```python
from build123d import *

# Parameters (mm, degrees)
F0_W     = 41
F0_H     = 41
F1_DEPTH = 4
F2_R     = 5


with BuildPart() as f1:
    # F0 (on Front) → F1 (new body)
    with BuildSketch(Plane.XZ):
        Rectangle(F0_W, F0_H)
        with BuildLine():
            ThreePointArc((-16, 14.3), (-17.202082, 17.202082), (-14.3, 16))
            Line((-14.3, 16), (-10.246951, 16))
            ThreePointArc((-10.246951, 16), (0, 19), (10.246951, 16))
            Line((10.246951, 16), (14.3, 16))
            ThreePointArc((14.3, 16), (16, 17.7), (17.7, 16))
            ThreePointArc((17.7, 16), (17.202082, 14.797918), (16, 14.3))
            Line((16, 14.3), (16, 10.246951))
            ThreePointArc((16, 10.246951), (18.234583, 5.338539), (19, 0))
            ThreePointArc((19, 0), (18.234583, -5.338539), (16, -10.246951))
            Line((16, -10.246951), (16, -14.3))
            ThreePointArc((16, -14.3), (17.202082, -14.797918), (17.7, -16))
            ThreePointArc((17.7, -16), (16, -17.7), (14.3, -16))
            Line((14.3, -16), (10.246951, -16))
            ThreePointArc((10.246951, -16), (0, -19), (-10.246951, -16))
            Line((-10.246951, -16), (-14.3, -16))
            ThreePointArc((-14.3, -16), (-17.202082, -17.202082), (-16, -14.3))
            Line((-16, -14.3), (-16, -10.246951))
            ThreePointArc((-16, -10.246951), (-19, 0), (-16, 10.246951))
            Line((-16, 10.246951), (-16, 14.3))
        make_face(mode=Mode.SUBTRACT)
    extrude(amount=F1_DEPTH)

    # F2
    f2_edges = [f1.edges().sort_by_distance(p)[0] for p in [
        (-20.5, -2, -20.5),
        (20.5, -2, -20.5),
        (20.5, -2, 20.5),
        (-20.5, -2, 20.5),
    ]]
    fillet(f2_edges, radius=F2_R)


solid = f1.part
```
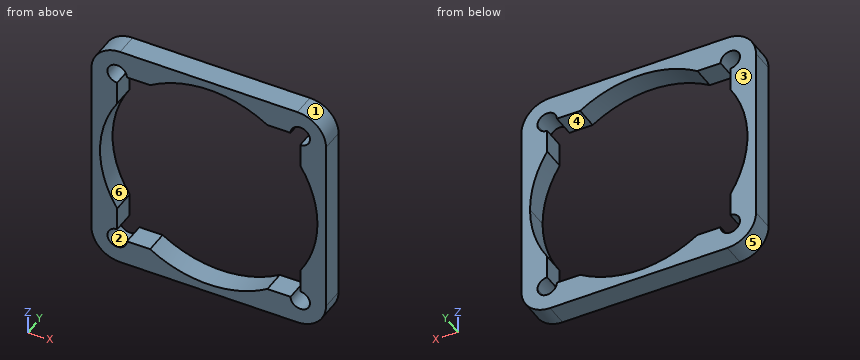
The model under review builds one solid part; all positions refer to its coordinate system, in mm. Face numbers are marked on the shaded views. A direction names the side the tool comes from. Round coordinates to 2 decimals unless told otherwise and drop trailing zeros. Write each loop counter-clockwise with the first axis right and the second up, starting at its lowest first coordinate (ties: lowest second). Pieces come first, ordered by that corner, then holes. Notation, with made-up numbers: M -30,-28 L -1,-28 A21 ccw -1,3 Z; hole C 43,-37 d3. An arc over 180 degrees is marked long. Use CSV: the item, a comma, the result in double quotes. Start each with the question number.
(1) We need section B-B, the plane x = -7.5. State the section outline as (y, z) points, then the cut area to 3 significant figures.
(2) Tool access review of the marked faces 5 and 6: name each direction out of +Z, -Z, +X, -X, +Y, -Y from which nothing blocks a thin tool from reaching the whole face with its end or side.
(3) We need section C-C, the plane z = 4. State the section outline as (x, y) points.
(4) The part is to be moulded in two halves that separate along Z. For the marked faces 1, 2, 3 and 4, say which applies: +Z half, -Z half, draft (parallel to the pull), parting line (faces both ways), or undercut.
(5) For line 1 along Z through (x, y) = (11.5, -1.8); line 2 along Z through (x, y) = (17, -1.05), list the stretches that pass through material, from the lowest coordinate up.
(6) We need section A-A, the plane y = -1.2. State the section outline as (x, z) points.
Findings:
1,outline,"M -4,-20.5 L 0,-20.5 L 0,-17.46 L -4,-17.46 Z; M -4,17.46 L 0,17.46 L 0,20.5 L -4,20.5 Z"
1,area,"24.3 mm^2"
2,face 5,"-Z, -X, +Y, -Y"
2,face 6,"+Y, -Y"
3,outline,"M -20.5,-4 L -18.57,-4 L -18.57,0 L -20.5,0 Z; M 18.57,-4 L 20.5,-4 L 20.5,0 L 18.57,0 Z"
4,face 1,"+Z half"
4,face 2,"undercut"
4,face 3,"draft"
4,face 4,"undercut"
5,line 1,"-20.5 to -16, 16 to 20.5"
5,line 2,"-20.27 to -17.37, -14.63 to -8.49, 8.49 to 14.63, 17.37 to 20.27"
6,outline,"M -20.5,-15.5 A5 ccw -15.5,-20.5 L 15.5,-20.5 A5 ccw 20.5,-15.5 L 20.5,15.5 A5 ccw 15.5,20.5 L -15.5,20.5 A5 ccw -20.5,15.5 Z; hole M -16,-14.3 A1.7 ccw long -14.3,-16 L -10.25,-16 A19 ccw 10.25,-16 L 14.3,-16 A1.7 ccw 17.7,-16 A1.7 ccw 16,-14.3 L 16,-10.25 A19 ccw 19,0 A19 ccw 16,10.25 L 16,14.3 A1.7 ccw 17.7,16 A1.7 ccw 14.3,16 L 10.25,16 A19 ccw -10.25,16 L -14.3,16 A1.7 ccw long -16,14.3 L -16,10.25 A19 ccw -16,-10.25 Z"
